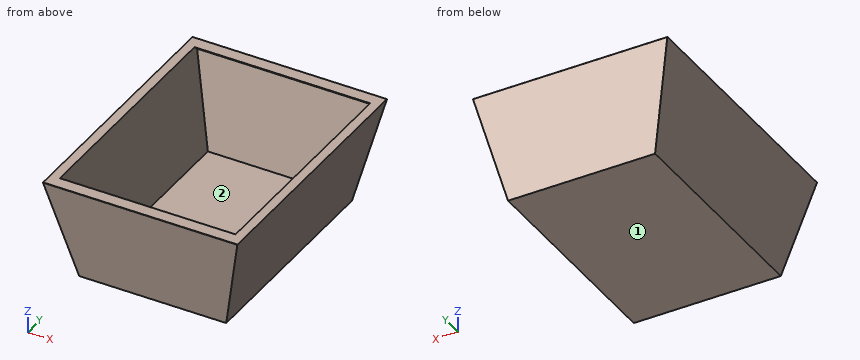
```python
from build123d import *

# Parameters (mm, degrees)
F0_W      = 16.1028504372
F0_H      = 24.0115216002
F2_W      = 24
F2_H      = 31
F5_W      = 14.02631565
F5_H      = 35.0832007825
F6_DEPTH  = 5
F8_W      = 36.7084983736
F8_H      = 15.6723505352
F9_DEPTH  = 5
F11_W     = 29.3105235323
F11_H     = 18.8404771034
F12_DEPTH = 5
F14_W     = 31.5226018429
F14_H     = 13.2806529291
F15_DEPTH = 5
F16_W     = 24.9057402834
F16_H     = 7.8468071297
F17_DEPTH = 25.4
F18_T     = -1


with BuildPart() as f3:
    # F0 (on Top) → F3 section 0
    with BuildSketch(Plane.XY):
        with Locations((0.0935448334, 0.0057467259)):
            Rectangle(F0_W, F0_H)
    # F2 (on offset) → F3 section 1
    with BuildSketch(Plane.XY.offset(17)):
        Rectangle(F2_W, F2_H)
    loft()

    # F5 (on face) → F6 (cut)
    with BuildSketch(Plane(origin=(-14.5, 0, 14.5), x_dir=(0.7071067812, 0, 0.7071067812), z_dir=(0.7071067812, 0, -0.7071067812))):
        with Locations((2.1269769641, -0.2655759454)):
            Rectangle(F5_W, F5_H)
    extrude(amount=F6_DEPTH, mode=Mode.SUBTRACT)

    # F8 (on face) → F9 (cut)
    with BuildSketch(Plane(origin=(14.5, 0, 14.5), x_dir=(0, 1, 0), z_dir=(0.7071067812, 0, 0.7071067812))):
        with Locations((-0.0566011295, 4.1208126349)):
            Rectangle(F8_W, F8_H)
    extrude(amount=-F9_DEPTH, mode=Mode.SUBTRACT)

    # F11 (on face) → F12 (cut)
    with BuildSketch(Plane(origin=(0, 16.25, 16.25), x_dir=(-1, 0, 0), z_dir=(0, 0.7071067812, 0.7071067812))):
        with Locations((0.3414950334, 3.7744397996)):
            Rectangle(F11_W, F11_H)
    extrude(amount=-F12_DEPTH, mode=Mode.SUBTRACT)

    # F14 (on face) → F15 (cut)
    with BuildSketch(Plane(origin=(0, -16.25, 16.25), x_dir=(1, 0, 0), z_dir=(0, 0.7071067812, -0.7071067812))):
        with Locations((0.8808970451, -0.6048630457)):
            Rectangle(F14_W, F14_H)
    extrude(amount=F15_DEPTH, mode=Mode.SUBTRACT)

    # F16 (on Front) → F17 (cut, symmetric)
    with BuildSketch(Plane.XZ):
        with Locations((-1.3808882795, 15.0799336843)):
            Rectangle(F16_W, F16_H)
    extrude(amount=F17_DEPTH, both=True, mode=Mode.SUBTRACT)

    # F18
    f18_openings = [f3.faces().sort_by_distance(p)[0] for p in [
        (0.032154, 0, 11.15653),
    ]]
    offset(amount=F18_T, openings=f18_openings)


solid = f3.part
```
Source: CAD feature listing. Evaluate the final solid. Frame: model axes, mm. Face numbers are marked on the shaded views. Give positions to 0.01 mm unless a question says otherwise; leave off trailing zeros.
1. Material intervals for line 1 along Y through (x, z) = (7.5, 2.5); line 2 along X through (y, z) = (6, 9.5); line 3 along Y through (x, z) = (-8.25, 6.25), sorted ascending.
2. First-contact query: pin 1 (1 mm diameter, centred on y = -10.5, z = 8, fed in from -X); pin 2 (2 mm diameter, centred on y = 0, z = 10, fed in from +X); pin 3 (1 mm diameter, centred on x = -2.5, y = 4, fed in from +Z). Flat tips, straight axial feed; report the tip coordinate or a pass-through.
3. Pull-direction query (Y, two-part tool) for the marked faces 1 and 2; classes: +Y half, -Y half, draft (parallel to the pull), parting line (faces both ways), or undercut.
Output values:
1. line 1: y = -12.51 to -11.49, 11.5 to 12.52
1. line 2: x = -10.22 to -9.19, 9.27 to 10.3
1. line 3: y = -13.29 to -12.27, 12.27 to 13.29
2. pin 1: stops at x = -9.98
2. pin 2: stops at x = 10.64
2. pin 3: stops at z = 1
3. face 1: draft
3. face 2: undercut
